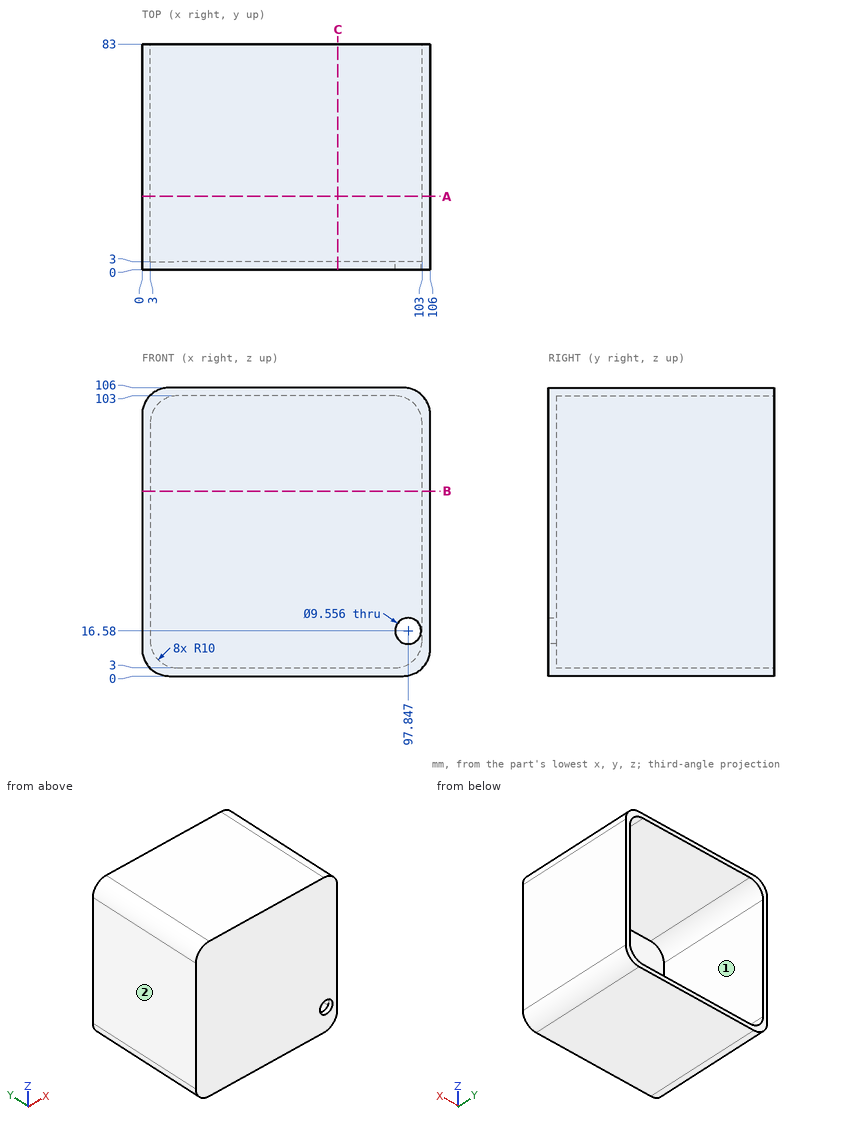
Here's the drawing with two shaded views (mm, measured from the low corner). I have some questions. A direction names the side the tool comes from. Coordinates: 2 decimals unless noted, no trailing zeros. Order: outer loops, then holes, each group sorted by start corner. A loop starts at its lowest first (then second) coordinate and runs counter-clockwise, first axis right, second up. Notation, with made-up numbers: (-27, 64.5) - (19, 64.5) arc R5 ccw to (19, 70.5) - close; hole circle Ø6 at (13, 21.5). An arc over 180 degrees is marked (long way). Use CSV: the item, a comma, the result in double quotes. Start each with the question number.
1. I'm going to push flat-ended pins straight in: pin 1 (5 mm diameter, centred on x = 49, z = 22, fed in from +Y); pin 2 (2 mm diameter, centred on x = 26.5, z = 65.5, fed in from -Y). Where does each tip first touch, or does it pass through?
2. Suppose I cut it at B-B on z = 68. List the corners of the cut face in (x, y) for me, then the cut area to 3 significant figures.
3. For the marked faces 1 and 2, which set-ups out of +Z, -Z, +X, -X, +Y, -Y let a thin tool reach every point of the face, with its end or its side?
4. Suppose I cut it at C-C on x = 72. List the corners of the cut face in (y, z) for me, then the cut area to 3 significant figures.
5. Please list where these lines run through material, in increasing order: line 1 (Z direction, x = 66, y = 57); line 2 (Y direction, x = 84, z = 31). Write a range as from..to.
6. Suppose I cut it at A-A on y = 27. List the corners of the cut face in (x, z) for me.
Output:
1,pin 1,"stops at y = 3"
1,pin 2,"stops at y = 0"
2,outline,"(0, 0) - (106, 0) - (106, 83) - (103, 83) - (103, 3) - (3, 3) - (3, 83) - (0, 83) - close"
2,area,"798 mm2"
3,face 1,"+Y"
3,face 2,"+Z, -Z, -X, +Y, -Y"
4,outline,"(0, 0) - (83, 0) - (83, 3) - (3, 3) - (3, 103) - (83, 103) - (83, 106) - (0, 106) - close"
4,area,"798 mm2"
5,line 1,"z = 0..3, 103..106"
5,line 2,"y = 0..3"
6,outline,"(0, 10) arc R10 ccw to (10, 0) - (96, 0) arc R10 ccw to (106, 10) - (106, 96) arc R10 ccw to (96, 106) - (10, 106) arc R10 ccw to (0, 96) - close; hole (3, 13) arc R10 ccw to (13, 3) - (93, 3) arc R10 ccw to (103, 13) - (103, 93) arc R10 ccw to (93, 103) - (13, 103) arc R10 ccw to (3, 93) - close"
